Could you check a few things on this drawing? It's one solid part, dimensions in mm from its lowest x, y, z. A direction names the side the tool comes from. Round coordinates to 2 decimals unless told otherwise and drop trailing zeros. Loops run counter-clockwise (first coordinate to the right, second up) from the corner with the lowest first, then second, coordinate; pieces in that order, holes last.
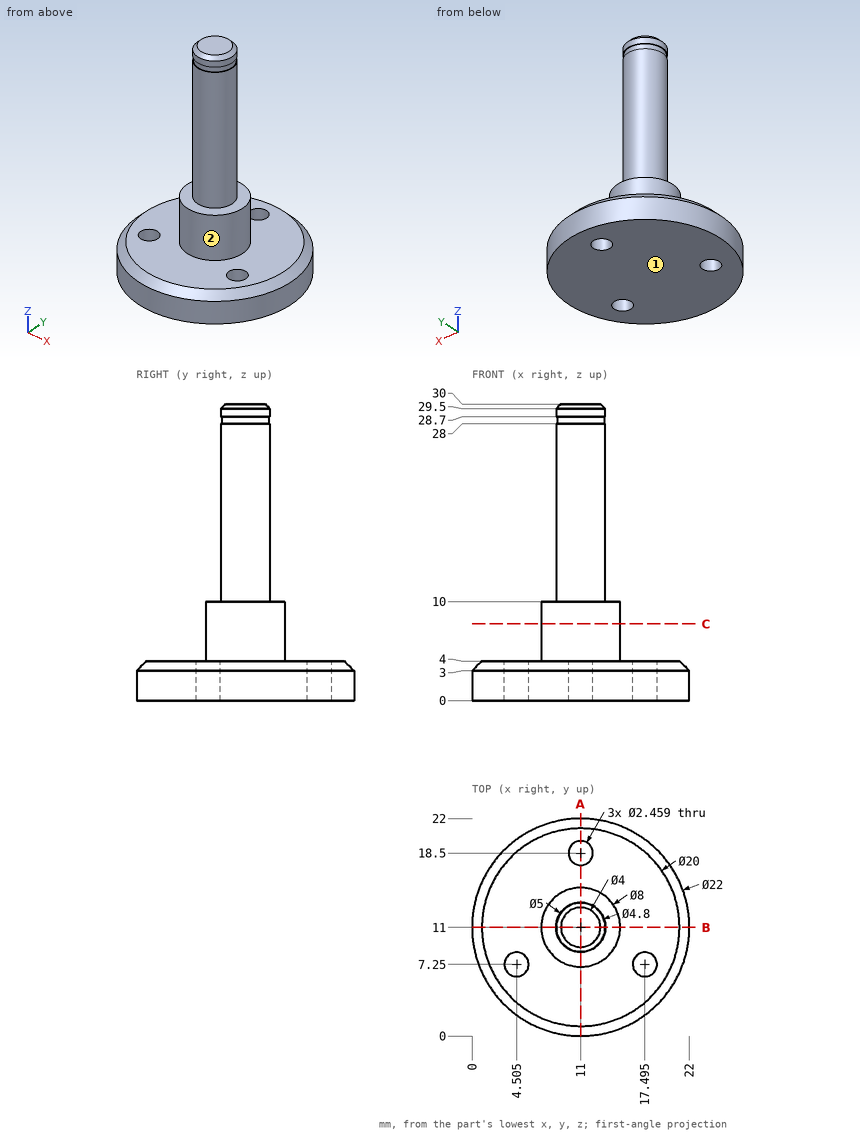
(1) If I drill on line 1 (X direction, y = 7.25, z = 2.4) (1 decimal); line 2 (Z direction, x = 13.5, y = 1.75); line 3 (X direction, y = 18, z = 2.5) (1 decimal), over which ranges is the centre line in solid material (lowest first)?
(2) Which directions (+Z, -Z, +X, -X, +Y, -Y) give clear straight access to the entire face, cutting with the end or side of a thin tool? Please do the marked faces 1 and 2.
(3) Suppose I cut it at C-C (z = 7.75). Write out the boundary of the cut face in (x, y).
(4) Suppose I cut it at A-A (x = 11). Write out the boundary of the cut face in (y, z), then the cut area to 3 significant figures.
(5) For pin 1 (4 mm diameter, centred on x = 11, y = 18.5, fed in from +Z); pin 2 (12 mm diameter, centred on y = 6.5, z = 13, fed in from -X); pin 3 (8 mm diameter, centred on y = 14.5, z = 21, fed in from +X), each with a flat end and sliding along its axis, tell me the tip position at first contact or that it passes through.
(6) Suppose I cut it at B-B (y = 11). Write out the boundary of the cut face in (x, z).
Check result:
1. line 1: x = 0.7 to 3.3, 5.7 to 16.3, 18.7 to 21.3
1. line 2: z = 0 to 4
1. line 3: x = 2.5 to 9.9, 12.1 to 19.5
2. face 1: -Z, +X, -X, +Y, -Y
2. face 2: +Z
3. outline: circle Ø8 at (11, 11)
4. outline: (0, 0) - (17.27, 0) - (17.27, 4) - (15, 4) - (15, 10) - (13.5, 10) - (13.5, 28) - (13.4, 28) - (13.4, 28.7) - (13.5, 28.7) - (13.5, 29.5) - (13, 30) - (9, 30) - (8.5, 29.5) - (8.5, 28.7) - (8.6, 28.7) - (8.6, 28) - (8.5, 28) - (8.5, 10) - (7, 10) - (7, 4) - (1, 4) - (0, 3) - close; (19.73, 0) - (22, 0) - (22, 3) - (21, 4) - (19.73, 4) - close
4. area: 225 mm2
5. pin 1: stops at z = 4
5. pin 2: stops at x = 7
5. pin 3: stops at x = 13.5
6. outline: (0, 0) - (22, 0) - (22, 3) - (21, 4) - (15, 4) - (15, 10) - (13.5, 10) - (13.5, 28) - (13.4, 28) - (13.4, 28.7) - (13.5, 28.7) - (13.5, 29.5) - (13, 30) - (9, 30) - (8.5, 29.5) - (8.5, 28.7) - (8.6, 28.7) - (8.6, 28) - (8.5, 28) - (8.5, 10) - (7, 10) - (7, 4) - (1, 4) - (0, 3) - close
